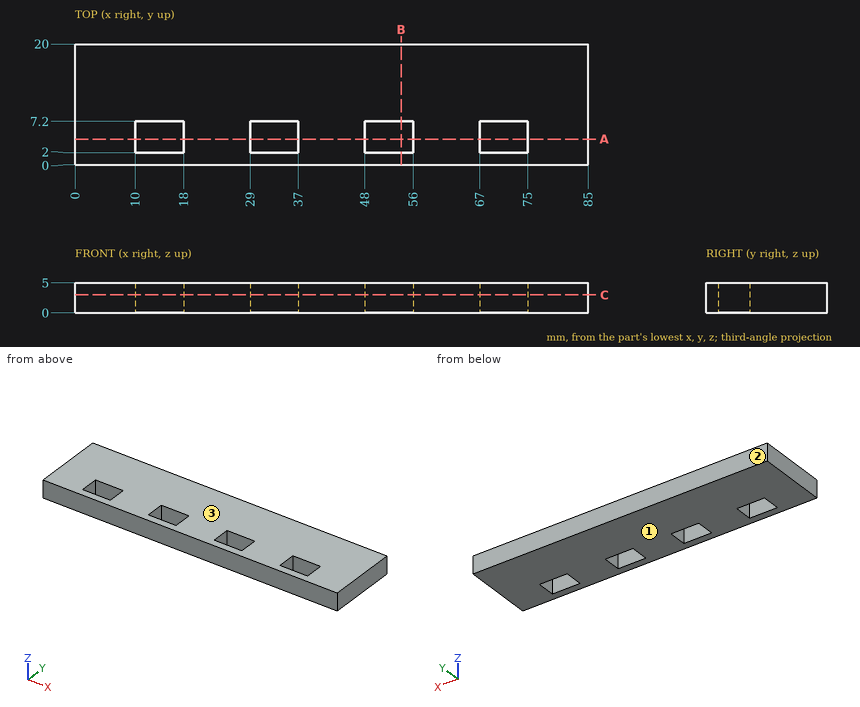
Geometry check sheet. Reference: drawing and pictorial views, mm from the part's lowest x, y, z. Coordinates: 2 decimals unless noted, no trailing zeros. Loops run counter-clockwise (first coordinate to the right, second up) from the corner with the lowest first, then second, coordinate; pieces in that order, holes last. Notation, with made-up numbers: (-29, 4.25) - (16, 4.25) arc R17 ccw to (16, 26.25) - close; hole circle Ø8 at (84.5, 60). An arc over 180 degrees is marked (long way). Return JSON: item names as keys, results as strings.
1. Section check A-A, the plane y = 4.25. Record the boundary of the cut face in (x, z).
Established:
{"outline": "(0, 0) - (10, 0) - (10, 5) - (0, 5) - close; (18, 0) - (29, 0) - (29, 5) - (18, 5) - close; (37, 0) - (48, 0) - (48, 5) - (37, 5) - close; (56, 0) - (67, 0) - (67, 5) - (56, 5) - close; (75, 0) - (85, 0) - (85, 5) - (75, 5) - close"}
2. Section check B-B, the plane x = 54. Record the boundary of the cut face in (y, z).
Established:
{"outline": "(0, 0) - (2, 0) - (2, 5) - (0, 5) - close; (7.2, 0) - (20, 0) - (20, 5) - (7.2, 5) - close"}
3. Mould release check, pull along Z, two halves, no side actions. Record for the marked faces 1, 2 and 3: +Z half, -Z half, draft (parallel to the pull), parting line (faces both ways), or undercut.
Established:
{"face 1": "-Z half", "face 2": "draft", "face 3": "+Z half"}
4. Section check C-C, the plane z = 3. Record the boundary of the cut face in (x, y).
Established:
{"outline": "(0, 0) - (85, 0) - (85, 20) - (0, 20) - close; hole (10, 2) - (18, 2) - (18, 7.2) - (10, 7.2) - close; hole (29, 2) - (37, 2) - (37, 7.2) - (29, 7.2) - close; hole (48, 2) - (56, 2) - (56, 7.2) - (48, 7.2) - close; hole (67, 2) - (75, 2) - (75, 7.2) - (67, 7.2) - close"}
5. Go/stop test with a flat-tipped pin: pin 1 (1 mm diameter, centred on x = 37, z = 2.5, fed in from -Y). Record where the tip stops, or that it passes through.
Established:
{"pin 1": "stops at y = 0"}
6. Thickness scan on L1, parallel to X at y = 2.75, z = 2.5; L2, parallel to Y at x = 71, z = 3.2. Record the ranges inside material, lowest first.
Established:
{"L1": "x = 0 to 10, 18 to 29, 37 to 48, 56 to 67, 75 to 85", "L2": "y = 0 to 2, 7.2 to 20"}
